Could you check a few things on this drawing? It's one solid part, dimensions in mm from its lowest x, y, z. A direction names the side the tool comes from. Give positions to 0.01 mm unless a question says otherwise; leave off trailing zeros. Loops run counter-clockwise (first coordinate to the right, second up) from the corner with the lowest first, then second, coordinate; pieces in that order, holes last. Notation, with made-up numbers: M -12.5,38.25 L 4.5,38.25 A22 cw 4.5,66.25 Z; hole C 84,-11.5 d1. An arc over 180 degrees is marked long. Answer as a JSON object with one key per item and string values.
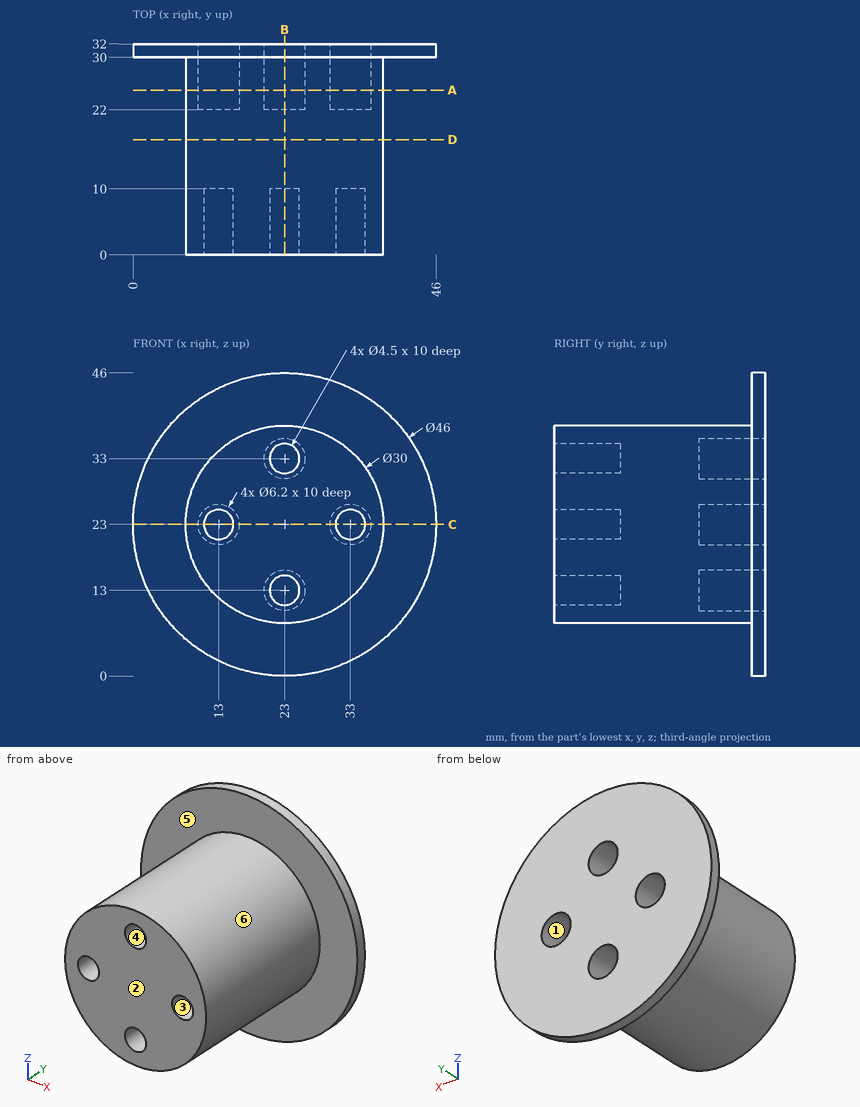
1) Suppose I cut it at D-D, the plane y = 17.5. Write out the boundary of the cut face in (x, z).
Answer list:
{"outline": "C 23,23 d30"}
2) Suppose I cut it at C-C, the plane z = 23. Write out the boundary of the cut face in (x, y).
Answer list:
{"outline": "M 0,30 L 8,30 L 8,0 L 10.75,0 L 10.75,10 L 15.25,10 L 15.25,0 L 30.75,0 L 30.75,10 L 35.25,10 L 35.25,0 L 38,0 L 38,30 L 46,30 L 46,32 L 36.1,32 L 36.1,22 L 29.9,22 L 29.9,32 L 16.1,32 L 16.1,22 L 9.9,22 L 9.9,32 L 0,32 Z"}
3) Will these pins go through, and if not, where does the flat tip stop? pin 1 Ø3.5 at (x, z) = (13, 23) entering from -Y; pin 2 Ø5 at (x, z) = (23, 33) entering from +Y; pin 3 Ø5 at (x, z) = (36.5, 41.5) entering from -Y.
Answer list:
{"pin 1": "y = 10", "pin 2": "y = 22", "pin 3": "y = 30"}
4) Please list where these lines run through material, in increasing order: line 1 along Z through (x, y) = (23, 6); line 2 along Z through (x, y) = (23, 29); line 3 along X through (y, z) = (5, 22.5). Write a range as from..to.
Answer list:
{"line 1": "8..10.75, 15.25..30.75, 35.25..38", "line 2": "8..9.9, 16.1..29.9, 36.1..38", "line 3": "8.01..10.81, 15.19..30.81, 35.19..37.99"}
5) For the marked faces 1, 2 and 3, which set-ups out of +Z, -Z, +X, -X, +Y, -Y let a thin tool reach every point of the face, with its end or its side?
Answer list:
{"face 1": "+Y", "face 2": "+Z, -Z, +X, -X, -Y", "face 3": "-Y"}
6) Suppose I cut it at A-A, the plane y = 25. Write out the boundary of the cut face in (x, z).
Answer list:
{"outline": "C 23,23 d30; hole C 13,23 d6.2; hole C 23,13 d6.2; hole C 23,33 d6.2; hole C 33,23 d6.2"}
7) If we mould it in two halves opening along X, with no side actions, what happens to the marked faces 4, 5 and 6? For each: +X half, -X half, draft (parallel to the pull), parting line (faces both ways), or undercut.
Answer list:
{"face 4": "undercut", "face 5": "draft", "face 6": "parting line"}
8) Suppose I cut it at B-B, the plane x = 23. Write out the boundary of the cut face in (y, z), and give its area (3 significant figures).
Answer list:
{"outline": "M 0,8 L 30,8 L 30,0 L 32,0 L 32,9.9 L 22,9.9 L 22,16.1 L 32,16.1 L 32,29.9 L 22,29.9 L 22,36.1 L 32,36.1 L 32,46 L 30,46 L 30,38 L 0,38 L 0,35.25 L 10,35.25 L 10,30.75 L 0,30.75 L 0,15.25 L 10,15.25 L 10,10.75 L 0,10.75 Z", "area": "778 mm^2"}
